```python
from build123d import *

# Parameters (mm, degrees)
SKETCH005_R       = 2.5
CYLINDER_R        = 11
CYLINDER_DEPTH    = 2
BOX001_W          = 26
BOX001_H          = 35
BOX001_DEPTH      = 26
CYLINDER001_R     = 1.5
CYLINDER001_DEPTH = 40
CYLINDER002_R     = 1.5
CYLINDER002_DEPTH = 40
BOX_W             = 4
BOX_H             = 12
BOX_DEPTH         = 12
CYLINDER003_R     = 3
CYLINDER003_DEPTH = 15
PAD_DEPTH         = 40
FILLET_R          = 2


with BuildPart() as sensorcable:
    # Sweep: sweep along a path in Sketch006
    with BuildLine(Plane.XY) as sweep_path:
        Line((20.046883, -0.001316), (20.046883, 39.998684))
        ThreePointArc((20.046883, 39.998684), (22.975815, 47.069752), (30.046883, 49.998684))
        Line((30.046883, 49.998684), (100.046883, 49.998684))
    # Sketch005 → Sweep (sweep)
    with BuildSketch(Plane.XZ):
        with Locations((20, 0.016)):
            Circle(SKETCH005_R)
    sweep(path=sweep_path.line)


with BuildPart() as sensorcable_1:
    # Sweep placement: moved
    add(sensorcable.part.moved(Location((0, 0, 20))))


with BuildPart() as sensorcylinder:
    # Cylinder → Cylinder (new body)
    with BuildSketch(Plane(origin=(20, 2, 20), x_dir=(1, 0, 0), z_dir=(0, -1, 0))):
        Circle(CYLINDER_R)
    extrude(amount=CYLINDER_DEPTH)


with BuildPart() as sensor:
    # Box001 → Box001 (new body)
    with BuildSketch(Plane(origin=(7, 2, 7), x_dir=(1, 0, 0), z_dir=(0, 0, 1))):
        with Locations((13, 17.5)):
            Rectangle(BOX001_W, BOX001_H)
    extrude(amount=BOX001_DEPTH)

    # Fusion001: union sensorCable, sensorCylinder
    add(sensorcable_1.part)
    add(sensorcylinder.part)


with BuildPart() as screw001:
    # Cylinder001 → Cylinder001 (new body)
    with BuildSketch(Plane(origin=(9, 51, 0), x_dir=(1, 0, 0), z_dir=(0, 0, 1))):
        Circle(CYLINDER001_R)
    extrude(amount=CYLINDER001_DEPTH)


with BuildPart() as screws:
    # Cylinder002 → Cylinder002 (new body)
    with BuildSketch(Plane(origin=(92, 9, 0), x_dir=(1, 0, 0), z_dir=(0, 0, 1))):
        Circle(CYLINDER002_R)
    extrude(amount=CYLINDER002_DEPTH)

    # Fusion002: union screw001
    add(screw001.part)


with BuildPart() as nutclamp:
    # Box → Box (new body)
    with BuildSketch(Plane(origin=(90, 20, 14), x_dir=(1, 0, 0), z_dir=(0, 0, 1))):
        with Locations((2, 6)):
            Rectangle(BOX_W, BOX_H)
    extrude(amount=BOX_DEPTH)


with BuildPart() as drills:
    # Cylinder003 → Cylinder003 (new body)
    with BuildSketch(Plane(origin=(85, 26, 20), x_dir=(0, 0, -1), z_dir=(1, 0, 0))):
        Circle(CYLINDER003_R)
    extrude(amount=CYLINDER003_DEPTH)

    # Fusion: union nutClamp
    add(nutclamp.part)

    # Fusion003: union sensor, screws
    add(sensor.part)
    add(screws.part)


with BuildPart() as ultrasonicsensorcase:
    # Sketch → Pad (new body)
    with BuildSketch(Plane.XY):
        Polygon((0, 0), (0, 60), (100, 60), (100, 0), (85, 0), (85, 40), (40, 40), (40, 0), align=None)
    extrude(amount=PAD_DEPTH)

    # Cut: cut drills
    add(drills.part, mode=Mode.SUBTRACT)

    # Fillet
    fillet_edges = [ultrasonicsensorcase.edges().sort_by_distance(p)[0] for p in [
        (0, 0, 20),
        (0, 60, 20),
        (40, 0, 20),
        (100, 60, 20),
        (40, 40, 20),
        (100, 0, 20),
        (85, 40, 20),
        (85, 0, 20),
    ]]
    fillet(fillet_edges, radius=FILLET_R)


solid = ultrasonicsensorcase.part
```
Can you work these out from the model? Positions are in its coordinate system, mm. A direction names the side the tool comes from. Round coordinates to 2 decimals unless told otherwise and drop trailing zeros. Loops run counter-clockwise (first coordinate to the right, second up) from the corner with the lowest first, then second, coordinate; pieces in that order, holes last. Notation, with made-up numbers: (-19.75, 66.25) -> (2.25, 66.25) arc R14 cw to (2.25, 90.25) -> close; hole circle Ø9 at (-16.75, -40). An arc over 180 degrees is marked (long way). Answer in a Markdown table with one row per item.
Item 1: Suppose I cut it at D-D, the plane z = 15. Give the number of separate pieces and of enclosed holes in the cut face, plus the area to 3 significant figures.
Answer block:
| item | result |
|---|---|
| separate pieces | 1 |
| enclosed holes | 3 |
| area | 3,190 mm² |
Item 2: Suppose I cut it at C-C, the plane y = 26. List the corners of the cut face in (x, z) for me.
Answer block:
| item | result |
|---|---|
| outline | (0, 0) -> (40, 0) -> (40, 40) -> (0, 40) -> close; (85, 0) -> (100, 0) -> (100, 17) -> (94, 17) -> (94, 14) -> (90, 14) -> (90, 17) -> (85, 17) -> close; (85, 23) -> (90, 23) -> (90, 26) -> (94, 26) -> (94, 23) -> (100, 23) -> (100, 40) -> (85, 40) -> close; hole (7, 7) -> (33, 7) -> (33, 33) -> (7, 33) -> close |
Item 3: Suppose I cut it at A-A, the plane y = 12.5. List the corners of the cut face in (x, z) for me, plus the area to 3 significant figures.
Answer block:
| item | result |
|---|---|
| outline | (0, 0) -> (40, 0) -> (40, 40) -> (0, 40) -> close; (85, 0) -> (100, 0) -> (100, 40) -> (85, 40) -> close; hole (7, 7) -> (33, 7) -> (33, 33) -> (7, 33) -> close |
| area | 1,520 mm² |
Item 4: We'd pull the mould along Y, two halves only. Please class faces 6 (the flat face through (7, 19, 20)), 7 (the cylindrical face through (0.57, 0.6, 20.28)), 8 (the flat face through (20, 20, 33)), 9 (the cylindrical face through (30.161, 1.014, 15.787)): released by +Y, released by -Y, zero draft, split by the parting line, or undercut.
Answer block:
| item | result |
|---|---|
| face 6 | undercut |
| face 7 | released by -Y |
| face 8 | undercut |
| face 9 | zero draft |
Item 5: Suppose I cut it at B-B, the plane z = 35. List the corners of the cut face in (x, y) for me.
Answer block:
| item | result |
|---|---|
| outline | (0, 2) arc R2 ccw to (2, 0) -> (38, 0) arc R2 ccw to (40, 2) -> (40, 38) arc R2 cw to (42, 40) -> (83, 40) arc R2 cw to (85, 38) -> (85, 2) arc R2 ccw to (87, 0) -> (98, 0) arc R2 ccw to (100, 2) -> (100, 58) arc R2 ccw to (98, 60) -> (2, 60) arc R2 ccw to (0, 58) -> close; hole circle Ø3 at (9, 51); hole circle Ø3 at (92, 9) |
Item 6: On a 3-axis mill with a long thin cutter (end or side, diameter ignored), from which of +Z, -Z, +X, -X, +Y, -Y can I reach the whole of each face in a straight line? I mean faces 1 (the cylindrical face through (87, 26, 23)), 2 (the cylindrical face through (8.675, 49.536, 19.72)), 3 (the cylindrical face through (99.4, 59.43, 20.28)), 4 (the flat face through (92, 26, 26)), 5 (the flat face through (40, 20, 20)). Say none if no direction works.
Answer block:
| item | result |
|---|---|
| face 1 | +X |
| face 2 | +Z, -Z |
| face 3 | +Z, -Z, +X, +Y |
| face 4 | none |
| face 5 | +Z, -Z, -Y |
Item 7: If I drill on probe 1 along X at (y, z) = (11.5, 25); probe 2 along Y at (x, z) = (87.45, 20); probe 3 along Z at (x, y) = (20, 1.5), over which ranges is the centre line in solid material (lowest first)?
Answer block:
| item | result |
|---|---|
| probe 1 | 0 to 7, 33 to 40, 85 to 100 |
| probe 2 | 0 to 23, 29 to 47.55, 52.55 to 60 |
| probe 3 | 0 to 9, 31 to 40 |
